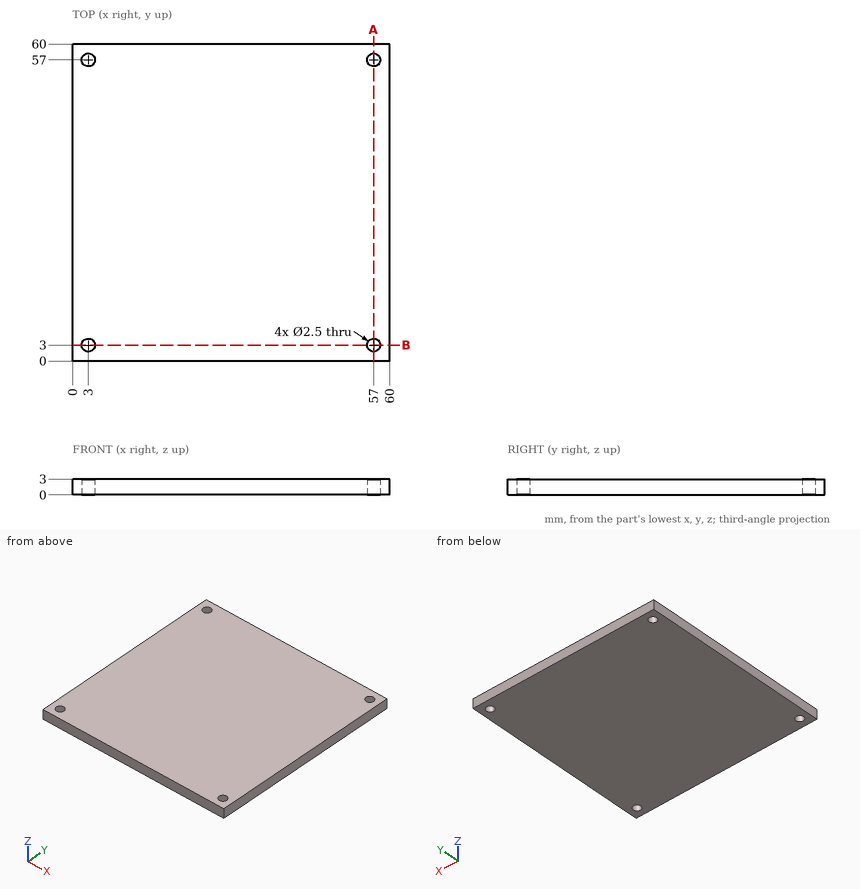
Can you work these out from the drawing? Everything is in mm from the part's minimum corner. Round coordinates to 2 decimals unless told otherwise and drop trailing zeros. Loops run counter-clockwise (first coordinate to the right, second up) from the corner with the lowest first, then second, coordinate; pieces in that order, holes last. Notation, with made-up numbers: (43.5, 43) - (59.5, 43) arc R31 cw to (59.5, 81) - close; hole circle Ø8 at (24.5, 10). An arc over 180 degrees is marked (long way). Answer in a Markdown table with one row per item. Add a question column.
Q1. I need wall thicknesses on L1, parallel to Y at x = 57, z = 1.3. Which ranges of the line are inside material? Lowest first, please.
Q2. I want a section at A-A on x = 57. List the corners of the cut face in (y, z) for me, and give its area (3 significant figures).
Q3. For pin 1 Ø2 at (x, y) = (3, 3) entering from +Z, with a flat end and sliding along its axis, tell me the tip position at first contact or that it passes through.
A:
| question | item | result |
|---|---|---|
| 1 | L1 | 0 to 1.75, 4.25 to 55.75, 58.25 to 60 |
| 2 | outline | (0, 0) - (1.75, 0) - (1.75, 3) - (0, 3) - close; (4.25, 0) - (55.75, 0) - (55.75, 3) - (4.25, 3) - close; (58.25, 0) - (60, 0) - (60, 3) - (58.25, 3) - close |
| 2 | area | 165 mm^2 |
| 3 | pin 1 | through |
